The listing builds one solid part. Answer for the finished solid, in the listing's coordinates (mm). A direction names the side the tool comes from. Give positions to 0.01 mm unless a question says otherwise; leave off trailing zeros. Order: outer loops, then holes, each group sorted by start corner. A loop starts at its lowest first (then second) coordinate and runs counter-clockwise, first axis right, second up. Notation, with made-up numbers: M 65,34 L 74,34 A26 ccw 74,69 Z; hole C 23,-7.5 d11. An arc over 180 degrees is marked long. Answer as a JSON object with one key per item and string values. Group by question number.
Autodesk Inventor part; units mm, degrees
ref_plane "bnt_s_1_XY" through (0, 0, 0) normal (-1, 0, 0) x (0, 0, -1)
ref_plane "bnt_s_1_YZ" through (0, 0, 0) normal (0, 0, -1) x (0, -1, 0)
ref_plane "bnt_s_1_ZX" through (0, 0, 0) normal (0, -1, 0) x (-1, 0, 0)
sketch "Sketch_1" plane through (0, 0, 0) normal (0, 0, 1) x (1, 0, 0)
  line L0 (341, 0) -> (5, 0)
  line L1 (5, 0) -> (5, 8)
  line L2 (5, 8) -> (341, 8)
  line L3 (341, 8) -> (341, 0)
  line L4 (341, 0) -> (5, 0)
revolve "Revolution1" add sketch "Sketch_1" angle 360 about axis through (341, 0, 0) along (1, 0, 0)
thread "Thread1"
sketch "Sketch_2" plane through (0, 0, 0) normal (0, 1, 0) x (-1, 0, 0)
  line L0 (-5, 0) -> (0, 0)
  line L1 (0, 0) -> (0, -7.2)
  line L2 (0, -7.2) -> (-0.8, -8)
  line L3 (-0.8, -8) -> (-4.8, -8)
  line L4 (-4.8, -8) -> (-4.8, -6.4)
  line L5 (-4.8, -6.4) -> (-5, -6.4)
  line L6 (-5, -6.4) -> (-5, 0)
  line L7 (-5, 0) -> (0, 0)
revolve "Revolution2" add sketch "Sketch_2" angle 360 about axis through (5, 0, 0) along (1, 0, 0)
sketch "Sketch_3" plane through (0, 0, 0) normal (0, 1, 0) x (-1, 0, 0)
  line L0 (-346, 0) -> (-341, 0)
  line L1 (-341, 0) -> (-341, -6.4)
  line L2 (-341, -6.4) -> (-341.2, -6.4)
  line L3 (-341.2, -6.4) -> (-341.2, -8)
  line L4 (-341.2, -8) -> (-345.2, -8)
  line L5 (-345.2, -8) -> (-346, -7.2)
  line L6 (-346, -7.2) -> (-346, 0)
  line L7 (-346, 0) -> (-341, 0)
revolve "Revolution3" add sketch "Sketch_3" angle 360 about axis through (346, 0, 0) along (1, 0, 0)
ref_plane "bnt_s_1_XY" through (0, 0, 0) normal (-1, 0, 0) x (0, 0, -1)
ref_plane "bnt_s_1_YZ" through (0, 0, 0) normal (0, 0, -1) x (0, -1, 0)
ref_plane "bnt_s_1_ZX" through (0, 0, 0) normal (0, -1, 0) x (-1, 0, 0)
properties part number "BNT 1605-2.6300 Shaft"
Item 1: Consider probe 1 along X at (y, z) = (6, 3); probe 2 along Y at (x, z) = (218, 0.5). Determine where each line is inside the solid, lowest interval first. Write a range as from..to.
Item 2: Section A-A (x = 87) is taken. Determine the outline of the cut face in (y, z).
Item 3: Flat-ended cylindrical pins translate along their axes: P1, Ø4, axis at x = 259.5, y = 6.5, coming from the +Z side; P2, Ø1, axis at x = 265.5, y = -6, coming from the +Z side; P3, Ø1.5, axis at x = 61, z = -6, coming from the -Y side. Find the tip coordinate at first contact, or state that the pin passes through.
Item 4: A tool of negligible diameter and unlimited length cuts with its end or side. For faces 1 (the flat face through (5, 0, 7)), 2 (the flat face through (0, 0, 0)), from which of +Z, -Z, +X, -X, +Y, -Y can it reach the whole face along a straight path? Write none if from no direction.
Values found:
{
 "1": {"probe 1": "x = 0..4.8, 5..341, 341.2..346", "probe 2": "y = -7.98..7.98"},
 "2": {"outline": "C 0,0 d16"},
 "3": {"P1": "stops at z = 6.61", "P2": "stops at z = 5.81", "P3": "stops at y = -6.04"},
 "4": {"face 1": "none", "face 2": "+Z, -Z, -X, +Y, -Y"}
}
